```python
from build123d import *

# Parameters (mm, degrees)
F2_W      = 51.3
F2_H      = 60.8
F2_R      = 1.8
F2_W_2    = 48.7926781061
F2_H_2    = 44.3010972813
F3_DEPTH  = 7
F4_DEPTH  = 15
F5_R      = 2.6
F6_DEPTH  = 25
F7_R      = 1.8
F8_DEPTH  = 2.6
F9_R      = 4.5
F9_R_2    = 2.6
F10_DEPTH = 6


with BuildPart() as f3:
    # F2 (on Top) → F3 (new body)
    with BuildSketch(Plane.XY):
        with Locations((25.65, -30.4)):
            Rectangle(F2_W, F2_H)
        with Locations((5.8, -55)):
            Circle(F2_R, mode=Mode.SUBTRACT)
        with Locations((47.3, -55)):
            Circle(F2_R, mode=Mode.SUBTRACT)
        with Locations((24.4784042297, -29.3142660521)):
            Rectangle(F2_W_2, F2_H_2, mode=Mode.SUBTRACT)
        with Locations((5.8, -4)):
            Circle(F2_R, mode=Mode.SUBTRACT)
        with Locations((47.3, -4)):
            Circle(F2_R, mode=Mode.SUBTRACT)
    extrude(amount=F3_DEPTH)

    # F4 (add): a face of the model
    f4_faces = [f3.faces().sort_by_distance(p)[0] for p in [
        (0, -30.4, 3.5),
    ]]
    extrude(f4_faces, amount=F4_DEPTH)

    # F5 (on face) → F6 (cut)
    with BuildSketch(Plane.XY.offset(7)):
        with Locations((-9.2740962282, -10)):
            Circle(F5_R)
        with Locations((-9.2740962282, -50.8)):
            Circle(F5_R)
    extrude(amount=-F6_DEPTH, mode=Mode.SUBTRACT)

    # F7 (on face) → F8 (cut)
    with BuildSketch(Plane(origin=(0, 0, 0), x_dir=(1, 0, 0), z_dir=(0, 0, -1))):
        Polygon((7.4743157806, 52.1), (9.1486315613, 55), (7.4743157806, 57.9), (4.1256842194, 57.9), (2.4513684387, 55), (4.1256842194, 52.1), align=None)
        with Locations((5.8, 55)):
            Circle(F7_R, mode=Mode.SUBTRACT)
        Polygon((48.9743157806, 52.1), (50.6486315613, 55), (48.9743157806, 57.9), (45.6256842194, 57.9), (43.9513684387, 55), (45.6256842194, 52.1), align=None)
        with Locations((47.3, 55)):
            Circle(F7_R, mode=Mode.SUBTRACT)
        Polygon((48.9743157806, 1.1), (50.6486315613, 4), (48.9743157806, 6.9), (45.6256842194, 6.9), (43.9513684387, 4), (45.6256842194, 1.1), align=None)
        with Locations((47.3, 4)):
            Circle(F7_R, mode=Mode.SUBTRACT)
        Polygon((7.4743157806, 1.1), (9.1486315613, 4), (7.4743157806, 6.9), (4.1256842194, 6.9), (2.4513684387, 4), (4.1256842194, 1.1), align=None)
        with Locations((5.8, 4)):
            Circle(F7_R, mode=Mode.SUBTRACT)
    extrude(amount=-F8_DEPTH, mode=Mode.SUBTRACT)

    # F9 (on face) → F10 (cut)
    with BuildSketch(Plane(origin=(0, 0, 0), x_dir=(1, 0, 0), z_dir=(0, 0, -1))):
        with Locations((-9.2740962282, 10)):
            Circle(F9_R)
        with Locations((-9.2740962282, 10)):
            Circle(F9_R_2, mode=Mode.SUBTRACT)
        with Locations((-9.2740962282, 50.8)):
            Circle(F9_R)
        with Locations((-9.2740962282, 50.8)):
            Circle(F9_R_2, mode=Mode.SUBTRACT)
    extrude(amount=-F10_DEPTH, mode=Mode.SUBTRACT)


solid = f3.part
```
Build history of the part. All positions in model axes, mm. A direction names the side the tool comes from. Coordinates: 2 decimals unless noted, no trailing zeros. Order: outer loops, then holes, each group sorted by start corner. A loop starts at its lowest first (then second) coordinate and runs counter-clockwise, first axis right, second up. Notation, with made-up numbers: (17, 69.25) -> (62, 69.25) arc R21 cw to (62, 106.25) -> close; hole circle Ø11 at (61, -34.5). An arc over 180 degrees is marked (long way). Answer in a Markdown table with one row per item. Add a question column.
Q1. Band-saw the part on A-A, the plane y = -24. List the corners of the cut face in (x, z), then the cut area to 3 significant figures.
Q2. Band-saw the part on C-C, the plane z = 0.75. Give the number of separate pieces and of enclosed holes in the cut face, then the cut area to 3 significant figures.
Q3. Mould opens along Y. For faces 3 (the face through (24, -7.164, 3)), 4 (the face through (19, -60.8, 3)), 5 (the face through (6, -57.9, 1)), 6 (the face through (-1, -26, 7)) say: +Y half, -Y half, draft (parallel to the pull), parting line (faces both ways), or undercut.
Q4. Band-saw the part on D-D, the plane x = 5.8. List the corners of the cut face in (y, z).
Q5. Drop flat-ended pins along their axis: pin 1 (3 mm diameter, centred on x = 47.3, y = -55, fed in from -Z) (3 decimals); pin 2 (4 mm diameter, centred on x = 5.8, y = -55, fed in from -Z); pin 3 (2.5 mm diameter, centred on x = -9, y = -8, fed in from -Z). Give the stop position or say it passes through.
Q6. Wall check: line 1 along X through (y, z) = (-50.8, 1.75); line 2 along Y through (x, z) = (47.3, 5.55); line 3 along Y through (x, z) = (1, 3.5). Give the ranges that are in metal, low to high. Write a range as [from, to].
Q7. Which spindle directions (+Z, -Z, +X, -X, +Y, -Y) get a long thin tool onto all of the face, cutting with end or side? Do faces 1 (the face through (49.8, -53.53, 1.28)), 2 (the face through (24, -51.465, 3)). Say none if no direction does.
Q8. Band-saw the part on B-B, the plane x = 20. List the corners of the cut face in (y, z).
Answers follow:
| question | item | result |
|---|---|---|
| 1 | outline | (-15, 0) -> (0.08, 0) -> (0.08, 7) -> (-15, 7) -> close; (48.87, 0) -> (51.3, 0) -> (51.3, 7) -> (48.87, 7) -> close |
| 1 | area | 123 mm^2 |
| 2 | separate pieces | 1 |
| 2 | enclosed holes | 7 |
| 2 | area | 1,630 mm^2 |
| 3 | face 3 | undercut |
| 3 | face 4 | -Y half |
| 3 | face 5 | undercut |
| 3 | face 6 | draft |
| 4 | outline | (-60.8, 0) -> (-57.9, 0) -> (-57.9, 2.6) -> (-56.8, 2.6) -> (-56.8, 7) -> (-60.8, 7) -> close; (-53.2, 2.6) -> (-52.1, 2.6) -> (-52.1, 0) -> (-51.46, 0) -> (-51.46, 7) -> (-53.2, 7) -> close; (-7.16, 0) -> (-6.9, 0) -> (-6.9, 2.6) -> (-5.8, 2.6) -> (-5.8, 7) -> (-7.16, 7) -> close; (-2.2, 2.6) -> (-1.1, 2.6) -> (-1.1, 0) -> (0, 0) -> (0, 7) -> (-2.2, 7) -> close |
| 5 | pin 1 | through |
| 5 | pin 2 | z = 2.6 |
| 5 | pin 3 | z = 6 |
| 6 | line 1 | [-15, -13.77], [-4.77, 0.08], [48.87, 51.3] |
| 6 | line 2 | [-60.8, -56.8], [-53.2, -51.46], [-7.16, -5.8], [-2.2, 0] |
| 6 | line 3 | [-60.8, -51.46], [-7.16, 0] |
| 7 | face 1 | -Z |
| 7 | face 2 | +Z, -Z |
| 8 | outline | (-60.8, 0) -> (-51.46, 0) -> (-51.46, 7) -> (-60.8, 7) -> close; (-7.16, 0) -> (0, 0) -> (0, 7) -> (-7.16, 7) -> close |
